from build123d import *

# Parameters (mm, degrees)
SKETCH1_R           = 1
BOSS_EXTRUDE1_DEPTH = 2
SKETCH2_R           = 4
SKETCH2_R_2         = 1
BOSS_EXTRUDE2_DEPTH = 6
CUT_EXTRUDE2_DEPTH  = 8
SKETCH5_W           = 3
SKETCH5_H           = 6
CUT_EXTRUDE3_DEPTH  = 16


with BuildPart() as part:
    # Sketch1 → Boss-Extrude1 (new body)
    with BuildSketch(Plane.XY):
        Polygon((-5, 3), (-3, 5), (3, 5), (5, 3), (5, -3), (3, -5), (-3, -5), (-5, -3), align=None)
        Circle(SKETCH1_R, mode=Mode.SUBTRACT)
    extrude(amount=BOSS_EXTRUDE1_DEPTH)

    # Sketch2 → Boss-Extrude2 (add)
    with BuildSketch(Plane.XY.offset(2)):
        Circle(SKETCH2_R)
        Circle(SKETCH2_R_2, mode=Mode.SUBTRACT)
    extrude(amount=BOSS_EXTRUDE2_DEPTH)

    # Sketch4 → Cut-Extrude2 (cut, symmetric)
    with BuildSketch(Plane(origin=(0, 0, 0), x_dir=(0, 0, -1), z_dir=(1, 0, 0))):
        Polygon((-8, -3), (-6.5, -3), (-6.5, 3), (-5, 3), (-5, 4), (-8, 4), align=None)
    extrude(amount=CUT_EXTRUDE2_DEPTH, both=True, mode=Mode.SUBTRACT)

    # Sketch5 → Cut-Extrude3 (cut)
    with BuildSketch(Plane(origin=(0, 0, 0), x_dir=(0, 0, -1), z_dir=(1, 0, 0))):
        with Locations((-5, 0)):
            Rectangle(SKETCH5_W, SKETCH5_H)
    extrude(amount=-CUT_EXTRUDE3_DEPTH, mode=Mode.SUBTRACT)


solid = part.part
Could you check a few things on this model? Use its own coordinates, in mm. A direction names the side the tool comes from. Give positions to 0.01 mm unless a question says otherwise; leave off trailing zeros. Order: outer loops, then holes, each group sorted by start corner. A loop starts at its lowest first (then second) coordinate and runs counter-clockwise, first axis right, second up.
1. Suppose I cut it at D-D (y = 1.5). List the corners of the cut face in (x, z) for me, plus the area to 3 significant figures.
2. We'd pull the mould along Y, two halves only. Please class faces 4 (the flat face through (1, 3, 6)), 5 (the flat face through (0, -2, 5)), 6 (the flat face through (0, 3.4, 5)): pulls with the +Y half, pulls with the -Y half, needs draft (parallel to the pull), parting line crosses it, or undercut.
3. Suppose I cut it at C-C (x = -3.5). List the corners of the cut face in (y, z) for me, plus the area to 3 significant figures.
4. I need wall thicknesses on L1, parallel to X at y = 0, z = 1.5; L2, parallel to Z at x = 3.5, y = -3.5. Which ranges of each line are inside material? Lowest first, please.
5. Suppose I cut it at A-A (y = 0). List the corners of the cut face in (x, z) for me.
6. For faces 1 (the flat face through (4.5, 0.1, 2)), 2 (the flat face through (2, 0, 6.5)), 3 (the flat face through (-1, -3, 6)), which set-ups out of +Z, -Z, +X, -X, +Y, -Y let a thin tool reach every point of the face, with its end or its side?
7. Will these pins go through, and if not, where does the flat tip stop? P1, Ø1, axis at x = 2, z = 6, coming from the -Y side; P2, Ø3, axis at x = 0, y = 0, coming from the +Z side; P3, Ø1.2, axis at x = -1.5, y = 0, coming from the +Z side; P4, Ø4.5, axis at x = 1.5, y = -1, coming from the +Z side.
8. Suppose I cut it at B-B (z = 5.5). List the corners of the cut face in (x, y) for me, plus the area to 3 significant figures.
Solved:
1. outline: (-5, 0) - (5, 0) - (5, 2) - (3.71, 2) - (3.71, 6.5) - (0, 6.5) - (0, 3.5) - (-3.71, 3.5) - (-3.71, 2) - (-5, 2) - close
1. area: 42.2 mm2
2. face 4: pulls with the +Y half
2. face 5: undercut
2. face 6: needs draft
3. outline: (-4.5, 0) - (4.5, 0) - (4.5, 2) - (1.94, 2) - (1.94, 3.5) - (-1.94, 3.5) - (-1.94, 2) - (-4.5, 2) - close
3. area: 23.8 mm2
4. L1: x = -5 to -1, 1 to 5
4. L2: z = 0 to 2
5. outline: (-5, 0) - (-1, 0) - (-1, 3.5) - (-4, 3.5) - (-4, 2) - (-5, 2) - close; (1, 0) - (5, 0) - (5, 2) - (4, 2) - (4, 6.5) - (1, 6.5) - close
6. face 1: +Z
6. face 2: +Z, +X, -X, +Y
6. face 3: +Z, -X
7. P1: stops at y = -3.71
7. P2: stops at z = 6.5
7. P3: stops at z = 3.5
7. P4: stops at z = 8
8. outline: (-2.65, -3) arc R4 ccw to (2.65, 3) - (0, 3) - (0, 1) arc R1 cw to (0, -1) - (0, -3) - close
8. area: 23.6 mm2
